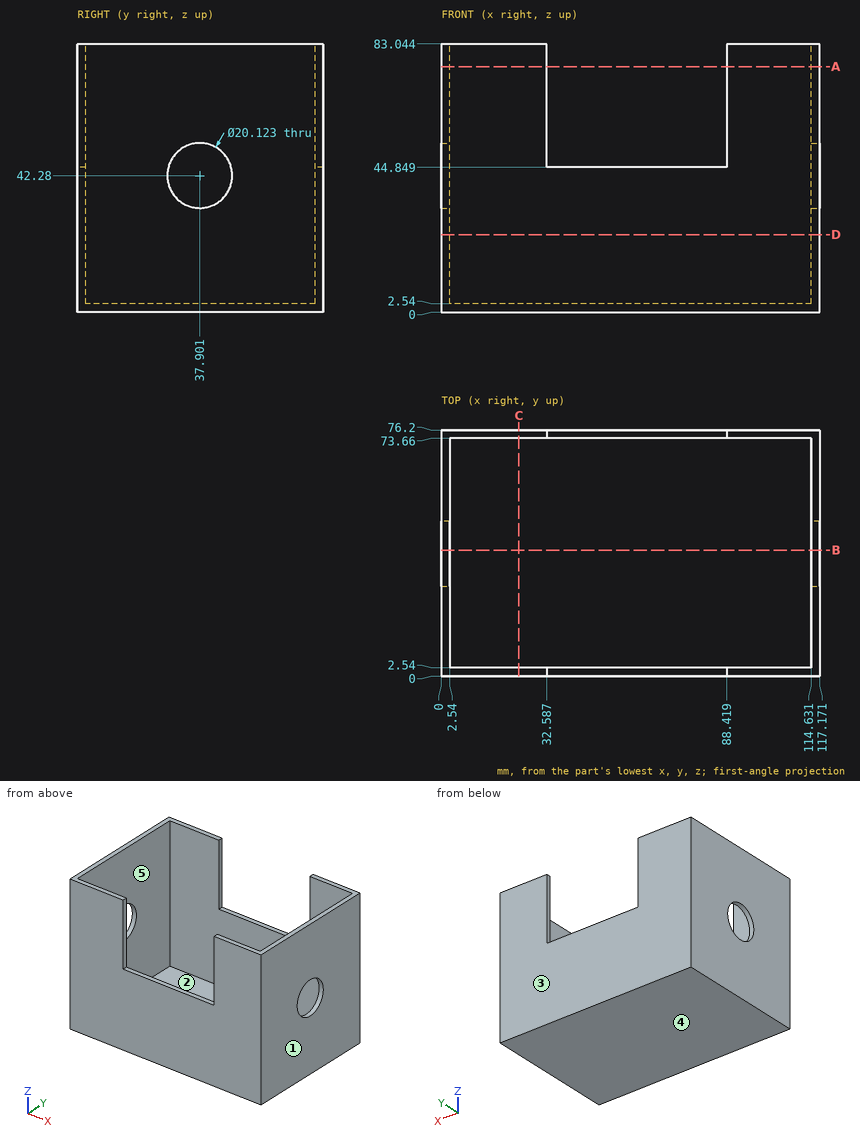
The figure shows three views and two pictorial views of one solid part (mm, origin at its lowest corner). Answer the questions. A direction names the side the tool comes from. Coordinates: 2 decimals unless noted, no trailing zeros. Loops run counter-clockwise (first coordinate to the right, second up) from the corner with the lowest first, then second, coordinate; pieces in that order, holes last. Notation, with made-up numbers: (85.25, 86) -> (103.25, 86) arc R25 cw to (103.25, 112) -> close; hole circle Ø7 at (75.25, 33.25). An arc over 180 degrees is marked (long way). Return JSON: item names as keys, results as strings. Group by question number.
(1) A cutting plane is placed at C-C on x = 24. Write down the section's boundary in (y, z).
(2) Determine the mould class of the marked faces 3, 4 and 5 for opening direction Y: released by +Y, released by -Y, zero draft, split by the parting line, or undercut.
(3) Given pin 1 Ø6 at (x, y) = (90.5, 25.5) entering from +Z; pin 2 Ø0.8 at (x, y) = (74, 1) entering from +Z, each flat-ended and moving along its own axis, determine where each tip first touches the part or whether it passes through.
(4) A cutting plane is placed at A-A on z = 76. Write down the section's boundary in (x, y).
(5) A cutting plane is placed at B-B on y = 39. Write down the section's boundary in (x, z).
(6) Find the intervals of material crossed by probe 1 along Y at (x, z) = (82.5, 33); probe 2 along X at (y, z) = (8, 74.5); probe 3 along Z at (x, y) = (24.5, 35), in increasing order. Write a range as from..to.
(7) A cutting plane is placed at D-D on z = 24. Write down the section's boundary in (x, y).
(8) Which of the six approach directions +Z, -Z, +X, -X, +Y, -Y give full straight-line access (tool end or side, diameter ignored) to the marked faces 1 and 2?
The answers:
{
 "1": {"outline": "(0, 0) -> (76.2, 0) -> (76.2, 83.04) -> (73.66, 83.04) -> (73.66, 2.54) -> (2.54, 2.54) -> (2.54, 83.04) -> (0, 83.04) -> close"},
 "2": {"face 3": "released by +Y", "face 4": "zero draft", "face 5": "undercut"},
 "3": {"pin 1": "stops at z = 2.54", "pin 2": "stops at z = 44.85"},
 "4": {"outline": "(0, 0) -> (32.59, 0) -> (32.59, 2.54) -> (2.54, 2.54) -> (2.54, 73.66) -> (32.59, 73.66) -> (32.59, 76.2) -> (0, 76.2) -> close; (88.42, 0) -> (117.17, 0) -> (117.17, 76.2) -> (88.42, 76.2) -> (88.42, 73.66) -> (114.63, 73.66) -> (114.63, 2.54) -> (88.42, 2.54) -> close"},
 "5": {"outline": "(0, 0) -> (117.17, 0) -> (117.17, 32.28) -> (114.63, 32.28) -> (114.63, 2.54) -> (2.54, 2.54) -> (2.54, 32.28) -> (0, 32.28) -> close; (0, 52.28) -> (2.54, 52.28) -> (2.54, 83.04) -> (0, 83.04) -> close; (114.63, 52.28) -> (117.17, 52.28) -> (117.17, 83.04) -> (114.63, 83.04) -> close"},
 "6": {"probe 1": "y = 0..2.54, 73.66..76.2", "probe 2": "x = 0..2.54, 114.63..117.17", "probe 3": "z = 0..2.54"},
 "7": {"outline": "(0, 0) -> (117.17, 0) -> (117.17, 76.2) -> (0, 76.2) -> close; hole (2.54, 2.54) -> (114.63, 2.54) -> (114.63, 73.66) -> (2.54, 73.66) -> close"},
 "8": {"face 1": "+Z, -Z, +X, +Y, -Y", "face 2": "+Z"}
}
